Here's how the part is built. I have some questions about the finished solid (model axes, mm). Face numbers are marked on the shaded views. A direction names the side the tool comes from. Round coordinates to 2 decimals unless told otherwise and drop trailing zeros. Write each loop counter-clockwise with the first axis right and the second up, starting at its lowest first coordinate (ties: lowest second). Pieces come first, ordered by that corner, then holes. Notation, with made-up numbers: M 68.5,52.5 L 122.5,52.5 A22 ccw 122.5,58.5 Z; hole C 12,-12.75 d11. An arc over 180 degrees is marked long. Use one line per item in the form item = value. Start each with the question number.
Q1. I want a section at A-A on y = 4.5. List the corners of the cut face in (x, z) for me, and give its area (3 significant figures).
Q2. For the marked faces 5 and 6, which set-ups out of +Z, -Z, +X, -X, +Y, -Y let a thin tool reach every point of the face, with its end or its side?
Q3. I want a section at B-B on z = 10.5. List the corners of the cut face in (x, y) for me.
Q4. We'd pull the mould along Z, two halves only. Please class the marked faces 1, 2, 3 and 4: +Z half, -Z half, draft (parallel to the pull), parting line (faces both ways), or undercut.
Q5. I want a section at C-C on x = 26.5. List the corners of the cut face in (y, z) for me, and give its area (3 significant figures).
Q6. I want a section at D-D on z = 2.5. List the corners of the cut face in (x, y) for me, and give its area (3 significant figures).
Q7. I need wall thicknesses on line 1 along X through (y, z) = (2.25, 3.5); line 2 along Z through (x, y) = (31.5, 2.25); line 3 along Y through (x, z) = (33.5, 11.5). Which ranges of each line are inside material? Lowest first, please. Write a range as from..to.
Q8. I'm going to push flat-ended pins straight in: pin 1 Ø0.9 at (x, y) = (-2, 4) entering from -Z; pin 2 Ø2 at (x, y) = (-1.5, 5.5) entering from +Z; pin 3 Ø0.5 at (y, z) = (5, 4) entering from -X; pin 4 Ø3 at (y, z) = (4.33, 9.56) entering from -X. Where does each tip first touch, or does it pass through?
```python
from build123d import *

# Parameters (mm, degrees)
F0_W        = 42.580999434
F0_H        = 7.9333577305
F1_DEPTH    = 13.97
F2_R        = 2.54
F3_DEPTH    = 45.0342
F4_T1_DEPTH = 20.6333577305
F4_T3_DEPTH = 55.280999434
F5_W        = 2.8782505542
F5_H        = 3.5978133092
F5_W_2      = 1.7989068292
F5_H_2      = 2.7433328796
F6_DEPTH    = 3.1496


# Not quite as in the source:
# - a fillet or chamfer that OpenCascade refuses, or shapes differently, is made with other operations: its cross-section is extruded or revolved along the edge and cut away or added


with BuildPart() as f1:
    # F0 (on Top) → F1 (new body)
    with BuildSketch(Plane.XY):
        with Locations((21.290499717, 3.9666788653)):
            Rectangle(F0_W, F0_H)
    extrude(amount=F1_DEPTH)

    # F2 (on Right) → F3 (cut)
    with BuildSketch(Plane.YZ):
        with Locations((4.3319589458, 9.5625361428)):
            Circle(F2_R)
    extrude(amount=F3_DEPTH, mode=Mode.SUBTRACT)

    # F4: fillet of radius 2.54 on 4 edges, made by hand

    # F4_s2 → F4_t1 (cut)
    with BuildSketch(Plane.XZ.offset(-14.2833577305)):
        with BuildLine():
            ThreePointArc((0, 11.43), (0.7439487758, 13.2260512242), (2.54, 13.97))
            Line((2.54, 13.97), (0, 13.97))
            Line((0, 13.97), (0, 11.43))
        make_face()
        with BuildLine():
            ThreePointArc((40.040999434, 13.97), (41.8370506582, 13.2260512242), (42.580999434, 11.43))
            Line((42.580999434, 11.43), (42.580999434, 13.97))
            Line((42.580999434, 13.97), (40.040999434, 13.97))
        make_face()
    extrude(amount=F4_T1_DEPTH, mode=Mode.SUBTRACT)

    # F4_s4 → F4_t3 (cut)
    with BuildSketch(Plane.YZ.offset(-6.35)):
        with BuildLine():
            ThreePointArc((7.9333577305, 11.43), (7.1894089547, 13.2260512242), (5.3933577305, 13.97))
            Line((5.3933577305, 13.97), (7.9333577305, 13.97))
            Line((7.9333577305, 13.97), (7.9333577305, 11.43))
        make_face()
        with BuildLine():
            ThreePointArc((2.54, 13.97), (0.7439487758, 13.2260512242), (0, 11.43))
            Line((0, 11.43), (0, 13.97))
            Line((0, 13.97), (2.54, 13.97))
        make_face()
    extrude(amount=F4_T3_DEPTH, mode=Mode.SUBTRACT)

    # F5 (on Right) → F6 (join)
    with BuildSketch(Plane.YZ):
        with Locations((4.8902533017, 3.1496292795)):
            Rectangle(F5_W, F5_H)
        with Locations((4.8902535345, 3.2170884078)):
            Rectangle(F5_W_2, F5_H_2, mode=Mode.SUBTRACT)
    extrude(amount=-F6_DEPTH)


solid = f1.part
```
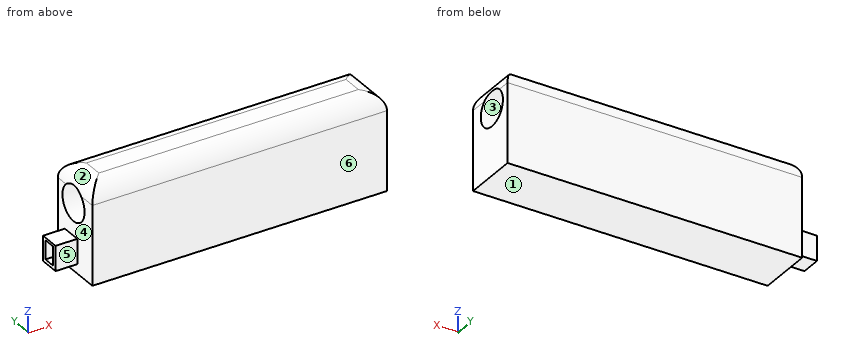
Reported:
q1.outline = M -3.15,1.35 L 0,1.35 L 0,0 L 42.58,0 L 42.58,7.03 L 0,7.03 L 0,4.95 L -3.15,4.95 L -3.15,4.59 L 0,4.59 L 0,1.85 L -3.15,1.85 Z; M 0.09,12.1 L 42.49,12.1 A2.54 ccw 40.04,13.97 L 2.54,13.97 A2.54 ccw Z
q1.area = 379 mm^2
q2.face_5 = +Z, -Z, -X, -Y
q2.face_6 = +Z, -Z, +X, -X, -Y
q3.outline = M 0,0 L 42.58,0 L 42.58,1.97 L 0,1.97 Z; M 0,6.69 L 42.58,6.69 L 42.58,7.93 L 0,7.93 Z
q4.face_1 = -Z half
q4.face_2 = +Z half
q4.face_3 = undercut
q4.face_4 = draft
q5.outline = M 0,0 L 7.93,0 L 7.93,11.43 A2.54 ccw 5.39,13.97 L 2.54,13.97 A2.54 ccw 0,11.43 Z; hole C 4.33,9.56 d5.08
q5.area = 87.8 mm^2
q6.outline = M -3.15,3.45 L 0,3.45 L 0,0 L 42.58,0 L 42.58,7.93 L 0,7.93 L 0,6.33 L -3.15,6.33 L -3.15,5.79 L 0,5.79 L 0,3.99 L -3.15,3.99 Z
q6.area = 341 mm^2
q7.line_1 = 0..42.58
q7.line_2 = 0..8.11, 11.02..13.95
q7.line_3 = 0..2.69, 5.97..7.93
q8.pin_1 = 1.35
q8.pin_2 = 4.95
q8.pin_3 = 0
q8.pin_4 = through
